Part model, mm, in its own coordinate system. A direction names the side the tool comes from. Round coordinates to 2 decimals unless told otherwise and drop trailing zeros. Loops run counter-clockwise (first coordinate to the right, second up) from the corner with the lowest first, then second, coordinate; pieces in that order, holes last. Notation, with made-up numbers: (56, 50.25) - (80, 50.25) arc R11 cw to (80, 64.25) - close; hole circle Ø5 at (39.5, 71). An arc over 180 degrees is marked (long way). Put each result on its own line as item: value.
Autodesk Inventor part; units mm, degrees
ref_plane "YZ Plane" through (0, 0, 0) normal (1, 0, 0) x (0, 1, 0)
ref_plane "XZ Plane" through (0, 0, 0) normal (0, 1, 0) x (-1, 0, 0)
ref_plane "XY Plane" through (0, 0, 0) normal (0, 0, 1) x (1, 0, 0)
sketch "Sketch1" plane through (0, 0, 0) normal (0, 1, 0) x (-1, 0, 0)
  circle A0 centre (0, 0) radius 5.15
  circle A1 centre (6.5, 0) radius 1
  circle A2 centre (3.25, 5.6292) radius 1
  circle A3 centre (-3.25, 5.6292) radius 1
  circle A4 centre (-6.5, 0) radius 1
  circle A5 centre (-3.25, -5.6292) radius 1
  circle A6 centre (3.25, -5.6292) radius 1
  line L0 (10, -18) -> (8, -18)
  line L1 (8, -18) -> (8, -20)
  line L2 (8, -20) -> (3, -20)
  line L3 (3, -20) -> (3, -18)
  line L4 (3, -18) -> (-3, -18)
  line L5 (-3, -18) -> (-3, -20)
  line L6 (-3, -20) -> (-8, -20)
  line L7 (-8, -20) -> (-8, -18)
  line L8 (-8, -18) -> (-10, -18)
  line L9 (10, -18) -> (10, 12)
  line L10 (-10, -18) -> (-10, 12)
  line L11 (10, 12) -> (8, 12)
  line L12 (8, 12) -> (8, 14)
  line L13 (8, 14) -> (3, 14)
  line L14 (3, 14) -> (3, 12)
  line L15 (3, 12) -> (-3, 12)
  line L16 (-3, 12) -> (-3, 14)
  line L17 (-3, 14) -> (-8, 14)
  line L18 (-8, 14) -> (-8, 12)
  line L19 (-8, 12) -> (-10, 12)
  dimension "d7" = 360
  dimension "d4" = 2
  dimension "d33" = 2
  dimension "d34" = 2
  dimension "d35" = 5
  dimension "d36" = 6
  dimension "d37" = 5
  dimension "d42" = 30
  dimension "d43" = 2
  dimension "d44" = 2
  dimension "d45" = 5
  dimension "d46" = 6
  dimension "d47" = 5
extrude "Extrusion1" add sketch "Sketch1" along normal blind 2
properties part number "Motor Mount"
1. Pin check, flat tips, straight feed: P1, Ø2.5, axis at x = 3.25, z = 5.63, coming from the +Y side; P2, Ø1, axis at y = 1, z = 13.5, coming from the -X side; P3, Ø1, axis at x = -9, y = 1.5, coming from the +Z side. Stop position of each tip, or through.
A:
P1: stops at y = 2
P2: stops at x = -8
P3: stops at z = 12
2. Band-saw the part on D-D (x = 6.5). List the corners of the cut face in (y, z), plus the area to 3 significant figures.
A:
outline: (0, -20) - (2, -20) - (2, -1) - (0, -1) - close; (0, 1) - (2, 1) - (2, 14) - (0, 14) - close
area: 64.0 mm²
3. Probe line 1 along Z through (x, y) = (0, 1.7); line 2 along Z through (x, y) = (3.25, 0.95) (3 decimals); line 3 along Z through (x, y) = (4, 0.45). List the from-to ranges inside material, lowest first. Write a range as [from, to].
A:
line 1: z = [-18, -5.15], [5.15, 12]
line 2: z = [-20, -6.629], [-4.629, -3.995], [3.995, 4.629], [6.629, 14]
line 3: z = [-20, -6.29], [-4.97, -3.24], [3.24, 4.97], [6.29, 14]
4. Two-plate mould, pull along X, no slides. Class faces 1 (the flat face through (0, 0, -7)), 2 (the flat face through (10, 1, -3)), 3 (the cylindrical face through (-2.25, 0.99, 5.59)), 4 (the flat face through (0, 1, 12)): pulls with the +X half, pulls with the -X half, needs draft (parallel to the pull), parting line crosses it, or undercut.
A:
face 1: needs draft
face 2: pulls with the +X half
face 3: undercut
face 4: undercut
5. Band-saw the part on A-A (z = 0). List the corners of the cut face in (x, y), plus the area to 3 significant figures.
A:
outline: (-10, 0) - (-7.5, 0) - (-7.5, 2) - (-10, 2) - close; (-5.5, 0) - (-5.15, 0) - (-5.15, 2) - (-5.5, 2) - close; (5.15, 0) - (5.5, 0) - (5.5, 2) - (5.15, 2) - close; (7.5, 0) - (10, 0) - (10, 2) - (7.5, 2) - close
area: 11.4 mm²
6. Tool access for faces 5 (the flat face through (0, 1, -18)), 6 (the flat face through (-9, 1, -18)), 7 (the flat face through (9, 1, -18)), 8 (the flat face through (-3, 1, 13)): list every direction of +Z, -Z, +X, -X, +Y, -Y with a clear straight run to the whole face (end or side of a thin tool).
A:
face 5: -Z, +Y, -Y
face 6: -Z, -X, +Y, -Y
face 7: -Z, +X, +Y, -Y
face 8: +Z, +Y, -Y
7. Band-saw the part on B-B (x = 0). List the corners of the cut face in (y, z).
A:
outline: (0, -18) - (2, -18) - (2, -5.15) - (0, -5.15) - close; (0, 5.15) - (2, 5.15) - (2, 12) - (0, 12) - close
8. Band-saw the part on C-C (y = 1.1). List the corners of the cut face in (x, z).
A:
outline: (-10, -18) - (-8, -18) - (-8, -20) - (-3, -20) - (-3, -18) - (3, -18) - (3, -20) - (8, -20) - (8, -18) - (10, -18) - (10, 12) - (8, 12) - (8, 14) - (3, 14) - (3, 12) - (-3, 12) - (-3, 14) - (-8, 14) - (-8, 12) - (-10, 12) - close; hole circle Ø2 at (-6.5, 0); hole circle Ø10.3 at (0, 0); hole circle Ø2 at (-3.25, -5.63); hole circle Ø2 at (-3.25, 5.63); hole circle Ø2 at (3.25, -5.63); hole circle Ø2 at (3.25, 5.63); hole circle Ø2 at (6.5, 0)
